CAD build for the part. Positions are in the model's coordinates, mm. A direction names the side the tool comes from. Round coordinates to 2 decimals unless told otherwise and drop trailing zeros. Loops run counter-clockwise (first coordinate to the right, second up) from the corner with the lowest first, then second, coordinate; pieces in that order, holes last. Notation, with made-up numbers: (-9, 76) -> (2, 76) arc R19 ccw to (2, 107) -> close; hole circle Ø3 at (38.5, 87). An arc over 180 degrees is marked (long way). Answer as CSV lines item,"result".
```python
from build123d import *

# Parameters (mm, degrees)
SKETCH1_W                                        = 130
SKETCH1_H                                        = 100
BOSS_EXTRUDE1_DEPTH                              = 65
SKETCH2_W                                        = 110
SKETCH2_H                                        = 80
CUT_EXTRUDE1_DEPTH                               = 10
CBORE_FOR_M6_HEX_HEAD_MACHINE_SCREW1_D           = 7
CBORE_FOR_M6_HEX_HEAD_MACHINE_SCREW1_CBORE_D     = 16
CBORE_FOR_M6_HEX_HEAD_MACHINE_SCREW1_CBORE_DEPTH = 4.7
SHELL1_START                                     = 15
SHELL1_OUTLINE_W                                 = 120
SHELL1_OUTLINE_H                                 = 95
SHELL1_OUTLINE_R                                 = 13
SHELL1_DEPTH                                     = 45
SHELL1_2_OUTLINE_R                               = 13
SHELL1_2_OUTLINE_R_2                             = 8.5
SHELL1_2_DEPTH                                   = 40.3
SHELL1_START_2                                   = -60
SHELL1_3_DEPTH                                   = 120
SHELL1_START_3                                   = -46
SHELL1_4_DEPTH                                   = 91
SKETCH6_R                                        = 4
SKETCH6_R_2                                      = 2.5
CUT_EXTRUDE2_DEPTH                               = 133.193040664


with BuildPart() as part:
    # Sketch1 → Boss-Extrude1 (new body)
    with BuildSketch(Plane(origin=(0, 0, 0), x_dir=(1, 0, 0), z_dir=(0, 1, 0))):
        Rectangle(SKETCH1_W, SKETCH1_H)
    extrude(amount=BOSS_EXTRUDE1_DEPTH)

    # Sketch2 → Cut-Extrude1 (cut)
    with BuildSketch(Plane.XZ):
        Rectangle(SKETCH2_W, SKETCH2_H)
    extrude(amount=-CUT_EXTRUDE1_DEPTH, mode=Mode.SUBTRACT)

    # Draft1: read off the stored shape, not the designer's step
    # Draft1: loft between two sections, ruled curve by curve
    draft1_from = [
        Edge.make_line((55, 10, -40), (-55, 10, -40)),
        Edge.make_line((-55, 10, -40), (-55, 10, 40)),
        Edge.make_line((-55, 10, 40), (55, 10, 40)),
        Edge.make_line((55, 10, 40), (55, 10, -40)),
    ]
    draft1_to = [
        Edge.make_line((58.639702343, 0, -43.639702343), (-58.639702343, 0, -43.639702343)),
        Edge.make_line((-58.639702343, 0, -43.639702343), (-58.639702343, 0, 43.639702343)),
        Edge.make_line((-58.639702343, 0, 43.639702343), (58.639702343, 0, 43.639702343)),
        Edge.make_line((58.639702343, 0, 43.639702343), (58.639702343, 0, -43.639702343)),
    ]
    draft1 = Solid(Shell([*[Face.make_surface_from_curves(draft1_from[k], draft1_to[k]) for k in range(4)], Face(Wire(draft1_from)), Face(Wire(draft1_to))]))
    add(draft1, mode=Mode.SUBTRACT)

    # CBORE for M6 Hex Head Machine Screw1 (through all)
    with Locations(Plane(origin=(0, 65, 0), x_dir=(1, 0, 0), z_dir=(0, 1, 0))):
        with Locations((0, 0)):
            CounterBoreHole(CBORE_FOR_M6_HEX_HEAD_MACHINE_SCREW1_D / 2, CBORE_FOR_M6_HEX_HEAD_MACHINE_SCREW1_CBORE_D / 2, CBORE_FOR_M6_HEX_HEAD_MACHINE_SCREW1_CBORE_DEPTH)

    # Shell1: read off the stored shape, not the designer's step
    # Shell1 outline → Shell1 (cut)
    with BuildSketch(Plane(origin=(0, 0, 0), x_dir=(1, 0, 0), z_dir=(0, 1, 0)).offset(SHELL1_START)):
        with Locations((0, 2.5)):
            Rectangle(SHELL1_OUTLINE_W, SHELL1_OUTLINE_H)
        Circle(SHELL1_OUTLINE_R, mode=Mode.SUBTRACT)
    extrude(amount=SHELL1_DEPTH, mode=Mode.SUBTRACT)

    # Shell1 2 outline → Shell1 2 (cut)
    with BuildSketch(Plane(origin=(0, 0, 0), x_dir=(1, 0, 0), z_dir=(0, 1, 0)).offset(SHELL1_START)):
        Circle(SHELL1_2_OUTLINE_R)
        Circle(SHELL1_2_OUTLINE_R_2, mode=Mode.SUBTRACT)
    extrude(amount=SHELL1_2_DEPTH, mode=Mode.SUBTRACT)

    # Shell1 3 outline → Shell1 3 (cut)
    with BuildSketch(Plane.YZ.offset(SHELL1_START_2)):
        Polygon((15, -43.501037691), (5, -47.140740034), (5, -50), (15, -50), align=None)
        Polygon((10.881634904, 45), (15, 43.501037691), (15, 45), align=None)
    extrude(amount=SHELL1_3_DEPTH, mode=Mode.SUBTRACT)

    # Shell1 4 outline → Shell1 4 (cut)
    with BuildSketch(Plane.XY.offset(SHELL1_START_3)):
        Polygon((-60, 15), (-60, 10.881634904), (-58.501037691, 15), align=None)
        Polygon((60, 15), (58.501037691, 15), (60, 10.881634904), align=None)
    extrude(amount=SHELL1_4_DEPTH, mode=Mode.SUBTRACT)

    # Sketch6 → Cut-Extrude2 (cut, through all)
    with BuildSketch(Plane(origin=(0, 0, 45), x_dir=(-1, 0, 0), z_dir=(0, 0, -1))):
        with Locations((-52, 23)):
            Circle(SKETCH6_R)
        with Locations((-52, 31)):
            Circle(SKETCH6_R_2)
        with Locations((-39, 31)):
            Circle(SKETCH6_R_2)
        with Locations((-39, 23)):
            Circle(SKETCH6_R)
        with Locations((-26, 31)):
            Circle(SKETCH6_R_2)
        with Locations((-26, 23)):
            Circle(SKETCH6_R)
        with Locations((-13, 31)):
            Circle(SKETCH6_R_2)
        with Locations((-13, 23)):
            Circle(SKETCH6_R)
        with Locations((0, 31)):
            Circle(SKETCH6_R_2)
        with Locations((0, 23)):
            Circle(SKETCH6_R)
        with Locations((13, 31)):
            Circle(SKETCH6_R_2)
        with Locations((13, 23)):
            Circle(SKETCH6_R)
        with Locations((26, 31)):
            Circle(SKETCH6_R_2)
        with Locations((26, 23)):
            Circle(SKETCH6_R)
        with Locations((39, 31)):
            Circle(SKETCH6_R_2)
        with Locations((39, 23)):
            Circle(SKETCH6_R)
        with Locations((52, 31)):
            Circle(SKETCH6_R_2)
        with Locations((52, 23)):
            Circle(SKETCH6_R)
    extrude(amount=-CUT_EXTRUDE2_DEPTH, mode=Mode.SUBTRACT)


solid = part.part
```
Q1. Slice it at C-C, the plane y = 13.5. Give the cut face in (x, z), and give its area (3 significant figures).
Results:
outline,"(-65, -50) -> (-60, -50) -> (-60, 45) -> (60, 45) -> (60, -50) -> (65, -50) -> (65, 50) -> (-65, 50) -> close; (-59.05, -44.05) -> (59.05, -44.05) -> (59.05, 44.05) -> (-59.05, 44.05) -> close; hole circle Ø7 at (0, 0)"
area,"12,000 mm2"
Q2. Slice it at B-B, the plane x = 39. Count the separate pieces of the cut face and the enclosed holes in it, and give its area (3 significant figures).
Results:
separate pieces,"3"
enclosed holes,"0"
area,"1,270 mm2"
Q3. Two-plate mould, pull along Z, no slides. Class faces 1 (the flat face through (-1, 39, 50)), 2 (the flat face through (-1, 35, 45)), 3 (the cylindrical face through (-40.34, 33.11, 47.46)): pulls with the +Z half, pulls with the -Z half, needs draft (parallel to the pull), parting line crosses it, or undercut.
Results:
face 1,"pulls with the +Z half"
face 2,"undercut"
face 3,"needs draft"
Q4. Probe L1, parallel to Y at x = -26, z = 47.25; L2, parallel to Y at x = -6, z = -18.5; L3, parallel to Z at x = -2, y = 45. List the from-to ranges inside material, lowest first. Write a range as [from, to].
Results:
L1,"[0, 19], [27, 28.5], [33.5, 65]"
L2,"[10, 15], [60, 65]"
L3,"[-8.26, -2.87], [2.87, 8.26], [45, 50]"
Q5. Tool access for faces 4 (the flat face through (-1, 5, -49)), 5 (the cylindrical face through (4.57, 34.868, -7.167)), 6 (the cylindrical face through (-1.34, 33.11, 47.46)): list every direction of +Z, -Z, +X, -X, +Y, -Y with a clear straight run to the whole face (end or side of a thin tool).
Results:
face 4,"-Z"
face 5,"none"
face 6,"+Z"
Q6. Slice it at A-A, the plane y = 36. Give the cut face in (x, z).
Results:
outline,"(-65, -50) -> (-60, -50) -> (-60, 45) -> (60, 45) -> (60, -50) -> (65, -50) -> (65, 50) -> (-65, 50) -> close; circle Ø17 at (0, 0); hole circle Ø7 at (0, 0)"
Q7. Drop flat-ended pins along their axis: pin 1 Ø9 at (x, y) = (-13, 23) entering from +Z; pin 2 Ø5 at (x, y) = (0, 23) entering from +Z; pin 3 Ø4 at (x, y) = (40, 8.5) entering from -Z; pin 4 Ø6.5 at (x, y) = (0, 31) entering from -Z. Give the stop position or say it passes through.
Results:
pin 1,"z = 50"
pin 2,"z = 8.5"
pin 3,"z = -46.59"
pin 4,"z = -8.5"
